The model under review builds one solid part; all positions refer to its coordinate system, in mm. Coordinates: 2 decimals unless noted, no trailing zeros. Write each loop counter-clockwise with the first axis right and the second up, starting at its lowest first coordinate (ties: lowest second). Pieces come first, ordered by that corner, then holes.
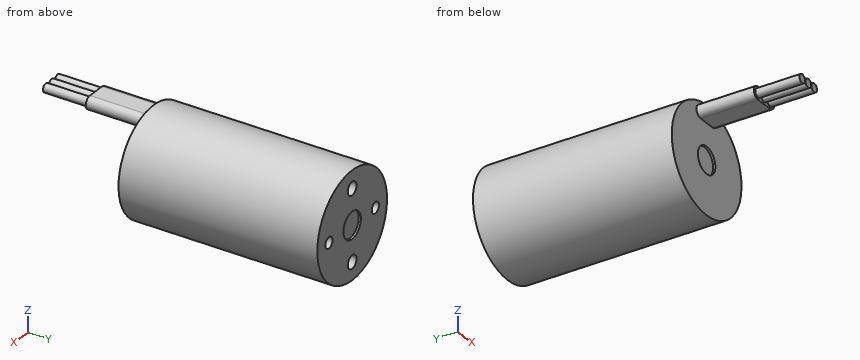
```python
from build123d import *

# Parameters (mm, degrees)
SKETCH1_R              = 12
MOTORCASE_DEPTH        = 45
HOLE_WIZARD_M2_5_D     = 2.5
HOLE_WIZARD_M2_5_DEPTH = 4
HOLE_WIZARD_M2_5_TIP   = 0.751075774
HOLE_WIZARD_M3_D       = 3
HOLE_WIZARD_M3_DEPTH   = 4
HOLE_WIZARD_M3_TIP     = 0.901290929
BOSS_EXTRUDE1_DEPTH    = 13
SKETCH15_R             = 0.966568062
BOSS_EXTRUDE2_DEPTH    = 10
SKETCH16_R             = 3
CUT_EXTRUDE2_DEPTH     = 0.5
CUT_EXTRUDE3_START     = -0.5
SKETCH17_R             = 3
CUT_EXTRUDE3_DEPTH     = 0.5


with BuildPart() as part:
    # Sketch1 → MotorCase (new body)
    with BuildSketch(Plane(origin=(0, 0, 0), x_dir=(1, 0, 0), z_dir=(0, 1, 0))):
        with Locations(Location((0, 0, 0), (0, 0, 90))):
            Circle(SKETCH1_R)
    extrude(amount=MOTORCASE_DEPTH)

    # Hole Wizard M2.5
    with Locations(Plane(origin=(0, 45, 0), x_dir=(1, 0, 0), z_dir=(0, 1, 0))):
        with Locations((8, 0), (-8, 0)):
            Hole(HOLE_WIZARD_M2_5_D / 2, depth=HOLE_WIZARD_M2_5_DEPTH)
            with Locations((0, 0, -(HOLE_WIZARD_M2_5_DEPTH + HOLE_WIZARD_M2_5_TIP / 2))):  # 118° drill point
                Cone(0, HOLE_WIZARD_M2_5_D / 2, HOLE_WIZARD_M2_5_TIP, mode=Mode.SUBTRACT)

    # Hole Wizard M3
    with Locations(Plane(origin=(0, 45, 0), x_dir=(1, 0, 0), z_dir=(0, 1, 0))):
        with Locations((0, 8), (0, -8)):
            Hole(HOLE_WIZARD_M3_D / 2, depth=HOLE_WIZARD_M3_DEPTH)
            with Locations((0, 0, -(HOLE_WIZARD_M3_DEPTH + HOLE_WIZARD_M3_TIP / 2))):  # 118° drill point
                Cone(0, HOLE_WIZARD_M3_D / 2, HOLE_WIZARD_M3_TIP, mode=Mode.SUBTRACT)

    # Sketch14 → Boss-Extrude1 (add)
    with BuildSketch(Plane.XZ):
        with BuildLine():
            Line((-2.053579932, 11), (2.053579932, 11))
            ThreePointArc((2.053579932, 11), (3.5, 9.553579932), (2.053579932, 8.107159865))
            Line((2.053579932, 8.107159865), (-2.053579932, 8.107159865))
            ThreePointArc((-2.053579932, 8.107159865), (-3.5, 9.553579932), (-2.053579932, 11))
        make_face()
    extrude(amount=BOSS_EXTRUDE1_DEPTH)

    # Sketch15 → Boss-Extrude2 (add)
    with BuildSketch(Plane.XZ.offset(13)):
        with Locations(Location((-2.053579932, 9.553579932, 0), (0, 0, 270))):
            Circle(SKETCH15_R)
        with Locations(Location((0, 9.553579932, 0), (0, 0, 270))):
            Circle(SKETCH15_R)
        with Locations(Location((2.053579932, 9.553579932, 0), (0, 0, 270))):
            Circle(SKETCH15_R)
    extrude(amount=BOSS_EXTRUDE2_DEPTH)

    # Sketch16 → Cut-Extrude2 (cut)
    with BuildSketch(Plane.XZ):
        with Locations(Location((0, 0, 0), (0, 0, 270))):
            Circle(SKETCH16_R)
    extrude(amount=-CUT_EXTRUDE2_DEPTH, mode=Mode.SUBTRACT)

    # Sketch17 → Cut-Extrude3 (cut)
    with BuildSketch(Plane(origin=(0, 45, 0), x_dir=(1, 0, 0), z_dir=(0, 1, 0)).offset(CUT_EXTRUDE3_START)):
        with Locations(Location((0, 0, 0), (0, 0, 90))):
            Circle(SKETCH17_R)
    extrude(amount=CUT_EXTRUDE3_DEPTH, mode=Mode.SUBTRACT)


solid = part.part
```
Item 1: To check wall thickness, follow line 1 along X through (y, z) = (0.1, 0); line 2 along Y through (x, z) = (4, -6.25); line 3 along X through (y, z) = (42.9, 8). State the ranges of each line that lie inside material, in increasing order.
Solved:
line 1: x = -12 to -3, 3 to 12
line 2: y = 0 to 45
line 3: x = -8.94 to -1.5, 1.5 to 8.94
Item 2: Take a section at B-B, the plane y = 15.5. Write out the cut boundary in (x, z).
Solved:
outline: circle Ø24 at (0, 0)
Item 3: Take a section at C-C, the plane z = -2. Write out the cut boundary in (x, y), plus the area to 3 significant figures.
Solved:
outline: (-11.83, 0) - (-2.24, 0) - (-2.24, 0.5) - (2.24, 0.5) - (2.24, 0) - (11.83, 0) - (11.83, 45) - (2.24, 45) - (2.24, 44.5) - (-2.24, 44.5) - (-2.24, 45) - (-11.83, 45) - close
area: 1,060 mm2
Item 4: For pin 1 (4 mm diameter, centred on x = -6.5, y = 8, fed in from +Z); pin 2 (1.8 mm diameter, centred on x = 0, z = 8, fed in from +Y); pin 3 (8 mm diameter, centred on x = 8.5, z = -9.5, fed in from +Y); pin 4 (1.5 mm diameter, centred on x = 3.5, y = 28, fed in from +Z), all flat-tipped, find the tip position at first contact; note any pin that passes through.
Solved:
pin 1: stops at z = 11.12
pin 2: stops at y = 40.64
pin 3: stops at y = 45
pin 4: stops at z = 11.68
Item 5: Take a section at A-A, the plane y = -15. Write out the cut boundary in (x, z), plus the area to 3 significant figures.
Solved:
outline: circle Ø1.93 at (-2.05, 9.55); circle Ø1.93 at (0, 9.55); circle Ø1.93 at (2.05, 9.55)
area: 8.81 mm2
